Part model, mm, in its own coordinate system. Face numbers are marked on the shaded views. A direction names the side the tool comes from. Give positions to 0.01 mm unless a question says otherwise; leave off trailing zeros. Order: outer loops, then holes, each group sorted by start corner. A loop starts at its lowest first (then second) coordinate and runs counter-clockwise, first axis right, second up. Notation, with made-up numbers: (7, -25) - (62, -25) arc R29 ccw to (62, -4) - close; hole circle Ø6 at (35.5, 48.5). An arc over 180 degrees is marked (long way). Use a Markdown table: item, result. Add a question column.
from build123d import *

# Parameters (mm, degrees)
SKETCH1_W                = 75
SKETCH1_H                = 35
BOSS_EXTRUDE1_DEPTH      = 5
SKETCH2_R                = 2
BOSS_EXTRUDE2_DEPTH      = 10
SKETCH3_W                = 75
SKETCH3_H                = 35
BOSS_EXTRUDE3_DEPTH      = 15
CUT_EXTRUDE2_DEPTH       = 10
SKETCH8_W                = 12.55
SKETCH8_H                = 5
SKETCH8_H_2              = 2.55
BOSS_EXTRUDE6_DEPTH      = 4.57
SKETCH9_R                = 2.1
CUT_EXTRUDE3_DEPTH       = 4.57
SKETCH14_W               = 3
SKETCH14_H               = 10
CUT_EXTRUDE5_DEPTH       = 17
SKETCH15_R               = 2.75
CUT_EXTRUDE6_DEPTH       = 1.5
FILLET1_R                = 1
CUT_EXTRUDE7_START       = -5
SKETCH19_R               = 2
CUT_EXTRUDE7_DEPTH       = 5
SKETCH20_W               = 6.17
SKETCH20_H               = 24
BOSS_EXTRUDE7_DEPTH      = 12
SKETCH21_W               = 6.17
SKETCH21_H               = 24
BOSS_EXTRUDE8_DEPTH      = 12
SKETCH24_R               = 2.1
CUT_EXTRUDE8_DEPTH       = 60.774520492
SKETCH25_R               = 4
CUT_EXTRUDE9_DEPTH       = 2
SKETCH26_W               = 3
SKETCH26_H               = 15
SKETCH26_H_2             = 6
BOSS_EXTRUDE9_DEPTH      = 8
SKETCH27_W               = 10.5
SKETCH27_H               = 4
CUT_EXTRUDE10_DEPTH      = 73.730684721
BOSS_EXTRUDE10_DEPTH     = 41
CUT_EXTRUDE11_DEPTH      = 100.332069343
CUT_EXTRUDE11_DEPTH_BACK = 100.332069343
SKETCH30_R               = 2.1
FILLET2_R                = 6.2


with BuildPart() as part:
    # Sketch1 → Boss-Extrude1 (new body)
    with BuildSketch(Plane.XY):
        Rectangle(SKETCH1_W, SKETCH1_H)
    extrude(amount=BOSS_EXTRUDE1_DEPTH)

    # Sketch2 → Boss-Extrude2 (add)
    with BuildSketch(Plane.XY.offset(5)):
        with Locations(Location((-14.2, 0.5, 0), (0, 0, 180))):
            Circle(SKETCH2_R)
        with Locations(Location((14.2, 0.5, 0), (0, 0, 180))):
            Circle(SKETCH2_R)
    extrude(amount=BOSS_EXTRUDE2_DEPTH)

    # Sketch3 → Boss-Extrude3 (add)
    with BuildSketch(Plane(origin=(0, 0, 0), x_dir=(-1, 0, 0), z_dir=(0, 0, -1))):
        Polygon((40.5, 20.5), (-37.5, 20.5), (-40.5, 20.5), (-40.5, -20.5), (40.5, -20.5), (40.5, -17.5), align=None)
        Rectangle(SKETCH3_W, SKETCH3_H, mode=Mode.SUBTRACT)
    extrude(amount=-BOSS_EXTRUDE3_DEPTH)

    # Sketch4 → Cut-Extrude2 (cut)
    with BuildSketch(Plane(origin=(0, 20.5, 0), x_dir=(1, 0, 0), z_dir=(0, 1, 0))):
        Polygon((-37.5, -5), (-37.5, -12.5), (-37.5, -14), (-37.5, -15), (37.5, -15), (37.5, -14), (37.5, -12.5), (37.5, -5), align=None)
    extrude(amount=-CUT_EXTRUDE2_DEPTH, mode=Mode.SUBTRACT)

    # Sketch8 → Boss-Extrude6 (add)
    with BuildSketch(Plane(origin=(0, 20.5, 0), x_dir=(1, 0, 0), z_dir=(0, 1, 0))):
        Polygon((0, -15), (0, -5), (-12.55, -5), (-12.55, -22.55), (0, -22.55), align=None)
        Polygon((12.55, -5), (0, -5), (0, -15), (0, -22.55), (12.55, -22.55), align=None)
        with Locations((-6.275, -2.5)):
            Rectangle(SKETCH8_W, SKETCH8_H)
        with Locations((-6.275, 1.275)):
            Rectangle(SKETCH8_W, SKETCH8_H_2)
        with Locations((6.275, 1.275)):
            Rectangle(SKETCH8_W, SKETCH8_H_2)
        with Locations((6.275, -2.5)):
            Rectangle(SKETCH8_W, SKETCH8_H)
    extrude(amount=BOSS_EXTRUDE6_DEPTH)

    # Sketch9 → Cut-Extrude3 (cut)
    with BuildSketch(Plane(origin=(0, 25.07, 0), x_dir=(1, 0, 0), z_dir=(0, 1, 0))):
        with Locations(Location((0, -10, 0), (0, 0, 270))):
            Circle(SKETCH9_R)
        with Locations(Location((-6.349818895, -3.650181105, 0), (0, 0, 270))):
            Circle(SKETCH9_R)
        with Locations(Location((6.349818895, -3.650181105, 0), (0, 0, 270))):
            Circle(SKETCH9_R)
        with Locations(Location((6.349818895, -16.349818895, 0), (0, 0, 270))):
            Circle(SKETCH9_R)
        with Locations(Location((-6.349818895, -16.349818895, 0), (0, 0, 270))):
            Circle(SKETCH9_R)
    extrude(amount=-CUT_EXTRUDE3_DEPTH, mode=Mode.SUBTRACT)

    # Sketch14 → Cut-Extrude5 (cut)
    with BuildSketch(Plane(origin=(0, 20.5, 0), x_dir=(1, 0, 0), z_dir=(0, 1, 0))):
        with Locations((-39, -10)):
            Rectangle(SKETCH14_W, SKETCH14_H)
        with Locations((39, -10)):
            Rectangle(SKETCH14_W, SKETCH14_H)
    extrude(amount=-CUT_EXTRUDE5_DEPTH, mode=Mode.SUBTRACT)

    # Sketch15 → Cut-Extrude6 (cut)
    with BuildSketch(Plane(origin=(0, 20.5, 0), x_dir=(1, 0, 0), z_dir=(0, 1, 0))):
        with Locations((-6.349818895, -3.650181105)):
            Circle(SKETCH15_R)
        with Locations((6.349818895, -3.650181105)):
            Circle(SKETCH15_R)
    extrude(amount=-CUT_EXTRUDE6_DEPTH, mode=Mode.SUBTRACT)

    # Fillet1
    fillet1_edges = [part.edges().sort_by_distance(p)[0] for p in [
        (-8.745750645, 19.75, 5),
        (-3.953887145, 19.75, 5),
        (3.953887145, 19.75, 5),
        (8.745750645, 19.75, 5),
    ]]
    fillet(fillet1_edges, radius=FILLET1_R)

    # Sketch19 → Cut-Extrude7 (cut)
    with BuildSketch(Plane.XY.offset(15).offset(CUT_EXTRUDE7_START)):
        with Locations(Location((-14.2, 0.5, 0), (0, 0, 180))):
            Circle(SKETCH19_R)
    extrude(amount=CUT_EXTRUDE7_DEPTH, mode=Mode.SUBTRACT)

    # Sketch20 → Boss-Extrude7 (add)
    with BuildSketch(Plane(origin=(40.5, 0, 0), x_dir=(0, 0, -1), z_dir=(1, 0, 0))):
        with Locations((-11.915, -8.5)):
            Rectangle(SKETCH20_W, SKETCH20_H)
    extrude(amount=BOSS_EXTRUDE7_DEPTH)

    # Sketch21 → Boss-Extrude8 (add)
    with BuildSketch(Plane.ZY.offset(40.5)):
        with Locations((11.915, -8.5)):
            Rectangle(SKETCH21_W, SKETCH21_H)
    extrude(amount=BOSS_EXTRUDE8_DEPTH)

    # Sketch24 → Cut-Extrude8 (cut, through all)
    with BuildSketch(Plane(origin=(0, 0, 8.83), x_dir=(-1, 0, 0), z_dir=(0, 0, -1))):
        with Locations(Location((-46.5, -3.5, 0), (0, 0, 90))):
            Circle(SKETCH24_R)
        with Locations(Location((-46.5, -13.5, 0), (0, 0, 90))):
            Circle(SKETCH24_R)
        with Locations(Location((46.5, -3.5, 0), (0, 0, 90))):
            Circle(SKETCH24_R)
        with Locations(Location((46.5, -13.5, 0), (0, 0, 90))):
            Circle(SKETCH24_R)
    extrude(amount=-CUT_EXTRUDE8_DEPTH, mode=Mode.SUBTRACT)

    # Sketch25 → Cut-Extrude9 (cut)
    with BuildSketch(Plane.XY.offset(15)):
        with Locations((-46.5, -3.5)):
            Circle(SKETCH25_R)
        with Locations((-46.5, -13.5)):
            Circle(SKETCH25_R)
        with Locations((46.5, -13.5)):
            Circle(SKETCH25_R)
        with Locations((46.5, -3.5)):
            Circle(SKETCH25_R)
    extrude(amount=-CUT_EXTRUDE9_DEPTH, mode=Mode.SUBTRACT)

    # Sketch26 → Boss-Extrude9 (add)
    with BuildSketch(Plane.XZ.offset(20.5)):
        with Locations((-9, 7.5)):
            Rectangle(SKETCH26_W, SKETCH26_H)
        with Locations((-9, 18)):
            Rectangle(SKETCH26_W, SKETCH26_H_2)
    extrude(amount=BOSS_EXTRUDE9_DEPTH)

    # Sketch27 → Cut-Extrude10 (cut, through all)
    with BuildSketch(Plane.ZY.offset(10.5)):
        with Locations((10.5, -24.5)):
            Rectangle(SKETCH27_W, SKETCH27_H)
    extrude(amount=-CUT_EXTRUDE10_DEPTH, mode=Mode.SUBTRACT)

    # Sketch28 → Boss-Extrude10 (add)
    with BuildSketch(Plane.XZ.offset(20.5)):
        Polygon((-25.5, 0), (-42.57, 0), (-42.57, -29.4), (-38, -29.4), (-38, -4), (-25.5, -4), align=None)
        Polygon((25.5, 0), (42.57, 0), (42.57, -29.4), (38, -29.4), (38, -4), (25.5, -4), align=None)
    extrude(amount=-BOSS_EXTRUDE10_DEPTH)

    # Sketch30 → Cut-Extrude11 (cut, two sides: drawn at the far end of the back side and taken through both)
    with BuildSketch(Plane(origin=(-38, 0, 0), x_dir=(0, 0, -1), z_dir=(1, 0, 0)).offset(-CUT_EXTRUDE11_DEPTH_BACK)):
        with Locations(Location((23.2, 0, 0), (0, 0, 180))):
            Circle(SKETCH30_R)
        with Locations(Location((23.2, 12.7, 0), (0, 0, 180))):
            Circle(SKETCH30_R)
        with Locations(Location((23.2, -12.7, 0), (0, 0, 180))):
            Circle(SKETCH30_R)
    extrude(amount=CUT_EXTRUDE11_DEPTH + CUT_EXTRUDE11_DEPTH_BACK, mode=Mode.SUBTRACT)

    # Fillet2
    # the kernel refuses this fillet: 6.2 mm, written as the material it takes off along each edge
    with BuildSketch(Plane(origin=(12.55, 5, 22.55), x_dir=(0, 0, -1), z_dir=(0, 1, 0))) as fillet2_piece_1:
        with BuildLine():
            CenterArc((FILLET2_R, FILLET2_R), FILLET2_R, 180, 90)
            Line((0, FILLET2_R), (0, 0))
            Line((0, 0), (FILLET2_R, 0))
        make_face()
    extrude(amount=35.57, mode=Mode.SUBTRACT)
    with BuildSketch(Plane(origin=(12.55, 20.5, -2.55), x_dir=(0, 0, 1), z_dir=(0, 1, 0))) as fillet2_piece_2:
        with BuildLine():
            CenterArc((FILLET2_R, -FILLET2_R), FILLET2_R, 90, 90)
            Line((0, -FILLET2_R), (0, 0))
            Line((0, 0), (FILLET2_R, 0))
        make_face()
    extrude(amount=20.07, mode=Mode.SUBTRACT)
    with BuildSketch(Plane(origin=(-12.55, 20.5, -2.55), x_dir=(0, 0, 1), z_dir=(0, 1, 0))) as fillet2_piece_3:
        with BuildLine():
            CenterArc((FILLET2_R, FILLET2_R), FILLET2_R, 180, 90)
            Line((0, FILLET2_R), (0, 0))
            Line((0, 0), (FILLET2_R, 0))
        make_face()
    extrude(amount=20.07, mode=Mode.SUBTRACT)
    with BuildSketch(Plane(origin=(-12.55, 5, 22.55), x_dir=(0, 0, -1), z_dir=(0, 1, 0))) as fillet2_piece_4:
        with BuildLine():
            CenterArc((FILLET2_R, -FILLET2_R), FILLET2_R, 90, 90)
            Line((0, -FILLET2_R), (0, 0))
            Line((0, 0), (FILLET2_R, 0))
        make_face()
    extrude(amount=35.57, mode=Mode.SUBTRACT)


solid = part.part
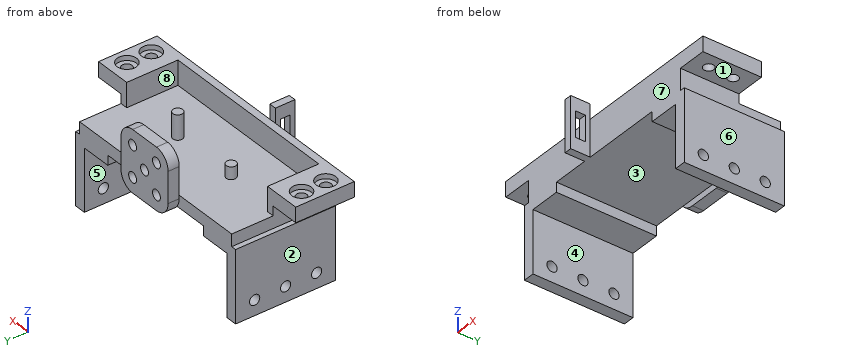
1. Tool access for the marked faces 5, 6, 7 and 8: list every direction of +Z, -Z, +X, -X, +Y, -Y with a clear straight run to the whole face (end or side of a thin tool).
2. Pin check, flat tips, straight feed: P1, Ø6, axis at y = -23, z = -22, coming from the +X side; P2, Ø2, axis at x = -14.5, y = 0.5, coming from the +Z side; P3, Ø1.4, axis at x = 1.5, y = 22, coming from the -Z side; P4, Ø2.5, axis at y = 12.7, z = -23.2, coming from the -X side. Stop position of each tip, or through.
3. Cut at D-D (z = -18). Write the cut outline in (x, y), plus the area to 3 significant figures.
4. Cut at A-A (z = -23.2). State how many separate pieces and enclosed holes the cut face has, plus the area to 3 significant figures.
5. Drill centre lines: probe 1 along Y at (x, z) = (41, -23); probe 2 along X at (y, z) = (-13, 12); probe 3 along Y at (x, z) = (-46, 11). Where is each one in solid material? Low to high. Write a range as [from, to].
6. Cut at C-C (y = 12.7). Write the cut outline in (x, z), plus the area to 3 significant figures.
7. Mould opens along X. For the marked faces 1, 2, 3 and 4 say: released by +X, released by -X, zero draft, split by the parting line, or undercut.
8. Cut at B-B (x = 46.5). Write the cut outline in (y, z), plus the area to 3 significant figures.
Responses:
| question | item | result |
|---|---|---|
| 1 | face 5 | -Z, +Y, -Y |
| 1 | face 6 | -Z, +X, +Y, -Y |
| 1 | face 7 | +Z, -Z, +X, -Y |
| 1 | face 8 | +Z, +Y |
| 2 | P1 | stops at x = 42.57 |
| 2 | P2 | stops at z = 10 |
| 2 | P3 | stops at z = -2.55 |
| 2 | P4 | passes through |
| 3 | outline | (-42.57, -20.5) - (-38, -20.5) - (-38, 20.5) - (-42.57, 20.5) - close; (38, -20.5) - (42.57, -20.5) - (42.57, 20.5) - (38, 20.5) - close |
| 3 | area | 375 mm² |
| 4 | separate pieces | 8 |
| 4 | enclosed holes | 0 |
| 4 | area | 260 mm² |
| 5 | probe 1 | y = [-20.5, -14.79], [-10.61, -2.09], [2.09, 10.61], [14.79, 20.5] |
| 5 | probe 2 | x = [-52.5, -48.54], [-44.46, -37.5], [37.5, 44.46], [48.54, 52.5] |
| 5 | probe 3 | y = [-20.5, -15.54], [-11.46, -5.54], [-1.46, 3.5] |
| 6 | outline | (-42.57, -29.4) - (-38, -29.4) - (-38, -25.3) - (-42.57, -25.3) - close; (-42.57, -21.1) - (-38, -21.1) - (-38, -4) - (-25.5, -4) - (-25.5, 0) - (25.5, 0) - (25.5, -4) - (38, -4) - (38, -21.1) - (42.57, -21.1) - (42.57, 0) - (40.5, 0) - (40.5, 5) - (-40.5, 5) - (-40.5, 0) - (-42.57, 0) - close; (38, -29.4) - (42.57, -29.4) - (42.57, -25.3) - (38, -25.3) - close |
| 6 | area | 735 mm² |
| 7 | face 1 | zero draft |
| 7 | face 2 | released by -X |
| 7 | face 3 | undercut |
| 7 | face 4 | undercut |
| 8 | outline | (-20.5, 8.83) - (-15.6, 8.83) - (-15.6, 13) - (-17.5, 13) - (-17.5, 15) - (-20.5, 15) - close; (-11.4, 8.83) - (-5.6, 8.83) - (-5.6, 13) - (-7.5, 13) - (-7.5, 15) - (-9.5, 15) - (-9.5, 13) - (-11.4, 13) - close; (-1.4, 8.83) - (3.5, 8.83) - (3.5, 15) - (0.5, 15) - (0.5, 13) - (-1.4, 13) - close |
| 8 | area | 81.1 mm² |
